Input: part model. Units: mm. Frame: model coordinates. Round coordinates to 2 decimals unless told otherwise and drop trailing zeros. Loops run counter-clockwise (first coordinate to the right, second up) from the corner with the lowest first, then second, coordinate; pieces in that order, holes last. Notation, with made-up numbers: (-6, -9) -> (8, -9) arc R6 ccw to (8, -4) -> close; hole circle Ø3 at (12, 89.5). An arc over 180 degrees is marked (long way). Answer as a JSON object with one key per item and string values.
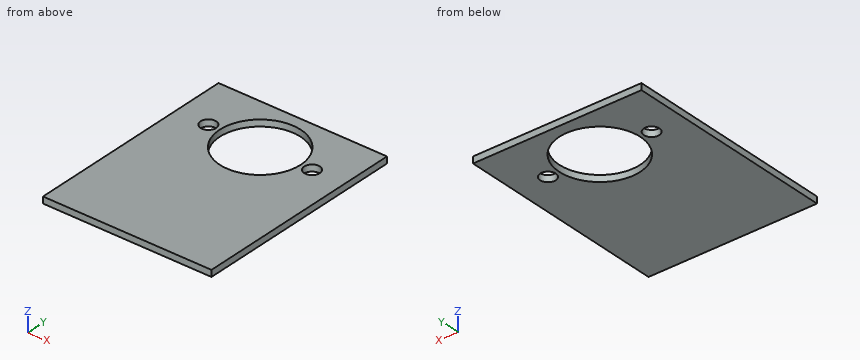
```python
from build123d import *

# Parameters (mm, degrees)
F0_W     = 82.55
F0_H     = 104.775
F1_DEPTH = 3.175
F2_R     = 19.812
F2_R_2   = 3.81
F3_DEPTH = 25.4


# Not quite as in the source:
# - a feature names something its author has since deleted; it is built from what else it names


with BuildPart() as f1:
    # F0 (on Top) → F1 (new body)
    with BuildSketch(Plane.XY):
        with Locations((0, -26.9875)):
            Rectangle(F0_W, F0_H)
    extrude(amount=F1_DEPTH)

    # F2 (on face) → F3 (cut)
    with BuildSketch(Plane.XY.offset(3.175)):
        Circle(F2_R)
        with Locations((-25.4, 0)):
            Circle(F2_R_2)
        with Locations((25.4, 0)):
            Circle(F2_R_2)
    extrude(amount=-F3_DEPTH, mode=Mode.SUBTRACT)


solid = f1.part
```
1) Section D-D, the plane y = -11. Output: boundary loops of the cut face in (x, z) (3 decimals).
Output:
{"outline": "(-41.275, 0) -> (-16.478, 0) -> (-16.478, 3.175) -> (-41.275, 3.175) -> close; (16.478, 0) -> (41.275, 0) -> (41.275, 3.175) -> (16.478, 3.175) -> close"}
2) Section C-C, the plane z = 2.2. Output: boundary loops of the cut face in (x, y) (3 decimals), plus the area to 3 significant figures.
Output:
{"outline": "(-41.275, -79.375) -> (41.275, -79.375) -> (41.275, 25.4) -> (-41.275, 25.4) -> close; hole circle Ø7.62 at (-25.4, 0); hole circle Ø39.624 at (0, 0); hole circle Ø7.62 at (25.4, 0)", "area": "7,320 mm^2"}
3) Ray query, probe 1 along Y at (x, z) = (25.4, 1.05) (3 decimals); probe 2 along Y at (x, z) = (0, 1.1) (3 decimals); probe 3 along X at (y, z) = (0.5, 0.7) (3 decimals). Return the intervals inside material, ascending.
Output:
{"probe 1": "y = -79.375 to -3.81, 3.81 to 25.4", "probe 2": "y = -79.375 to -19.812, 19.812 to 25.4", "probe 3": "x = -41.275 to -29.177, -21.623 to -19.806, 19.806 to 21.623, 29.177 to 41.275"}
4) Section A-A, the plane x = -25.4. Output: boundary loops of the cut face in (y, z) (3 decimals), plus the area to 3 significant figures.
Output:
{"outline": "(-79.375, 0) -> (-3.81, 0) -> (-3.81, 3.175) -> (-79.375, 3.175) -> close; (3.81, 0) -> (25.4, 0) -> (25.4, 3.175) -> (3.81, 3.175) -> close", "area": "308 mm^2"}
5) Section B-B, the plane y = 0. Output: boundary loops of the cut face in (x, z) (3 decimals), plus the area to 3 significant figures.
Output:
{"outline": "(-41.275, 0) -> (-29.21, 0) -> (-29.21, 3.175) -> (-41.275, 3.175) -> close; (-21.59, 0) -> (-19.812, 0) -> (-19.812, 3.175) -> (-21.59, 3.175) -> close; (19.812, 0) -> (21.59, 0) -> (21.59, 3.175) -> (19.812, 3.175) -> close; (29.21, 0) -> (41.275, 0) -> (41.275, 3.175) -> (29.21, 3.175) -> close", "area": "87.9 mm^2"}
6) Contact query for a flat-ended pin moving along its axis: P1, Ø10, axis at x = -25.4, y = 0, coming from the -Z side. Output: stop coordinate, or through.
Output:
{"P1": "stops at z = 0"}
